```python
from build123d import *

# Parameters (mm, degrees)
CROSSRECESS_DEPTH = 2.17
FILLET5_R         = 0.3
DRAFT1_ANGLE      = -30


with BuildPart() as part:
    # Sketch1 → Base (revolve)
    with BuildSketch(Plane.XY, mode=Mode.PRIVATE) as base_sk:
        with BuildLine():
            Line((11.1, 2), (4.5, 2))
            Line((4.5, 2), (3.1, 2))
            Line((3.1, 2), (3.1, 2.35))
            Line((3.1, 2.35), (3.1, 4))
            Line((3.1, 4), (1.376524617, 4))
            ThreePointArc((1.376524617, 4), (0.353757652, 2.115113473), (0, 0))
            Line((0, 0), (11.1, 0))
            Line((11.1, 0), (11.1, 2))
        make_face()
    revolve(base_sk.sketch.rotate(Axis((4.515812911, 0, 0), (-1, 0, 0)), 90), axis=Axis((4.515812911, 0, 0), (-1, 0, 0)))

    # Sketch6 → CrossRecess (cut)
    with BuildSketch(Plane(origin=(0, 0, 0), x_dir=(0, 0, -1), z_dir=(1, 0, 0))):
        Polygon((0.44, 0.44), (0.44, 2.2), (-0.44, 2.2), (-0.44, 0.44), (-2.2, 0.44), (-2.2, -0.44), (-0.44, -0.44), (-0.44, -2.2), (0.44, -2.2), (0.44, -0.44), (2.2, -0.44), (2.2, 0.44), align=None)
    extrude(amount=CROSSRECESS_DEPTH, mode=Mode.SUBTRACT)

    # Fillet5
    fillet5_edges = [part.edges().sort_by_distance(p)[0] for p in [
        (1.099926585, 0.44, 0.44),
        (1.099926585, -0.44, 0.44),
        (1.099926585, -0.44, -0.44),
        (1.099926585, 0.44, -0.44),
    ]]
    fillet(fillet5_edges, radius=FILLET5_R)

    # Draft1
    draft1_faces = [part.faces().sort_by_distance(p)[0] for p in [
        (1.27944778, -2.2, 0),
        (1.27944778, 0, -2.2),
        (1.27944778, 0, 2.2),
        (1.27944778, 2.2, 0),
    ]]
    draft(draft1_faces, Plane(origin=(0, 0, 0), x_dir=(0, 0, 1), z_dir=(1, 0, 0)), DRAFT1_ANGLE)


solid = part.part
```
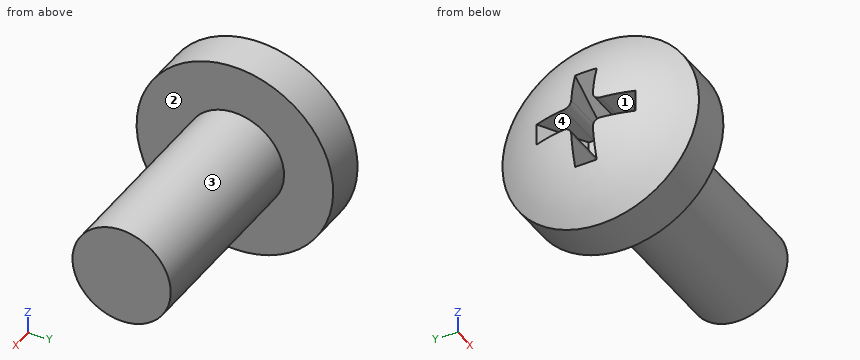
Can you work these out from the model? Positions are in its coordinate system, mm. Face numbers are marked on the shaded views. Give positions to 0.01 mm unless a question says otherwise; leave off trailing zeros. Order: outer loops, then holes, each group sorted by start corner. A loop starts at its lowest first (then second) coordinate and runs counter-clockwise, first axis right, second up. Notation, with made-up numbers: M 50.5,-12.5 L 84.5,-12.5 A24 ccw 84.5,19.5 Z; hole C -7,33 d4. An arc over 180 degrees is marked long. Write item = value, one per line. Start each with the question number.
Q1. I need wall thicknesses on probe 1 along Y at (x, z) = (7.5, 0); probe 2 along X at (y, z) = (0.5, 0); probe 3 along Z at (x, y) = (1.25, 0.5). Which ranges of each line are inside material? Lowest first, please. Write a range as [from, to].
Q2. Will these pins go through, and if not, where does the flat tip stop? pin 1 Ø1.5 at (y, z) = (3, 3) entering from +X; pin 2 Ø3 at (y, z) = (1.5, -2.5) entering from -X; pin 3 Ø0.6 at (y, z) = (-0.5, 0.5) entering from -X; pin 4 Ø1 at (x, z) = (1, 1.5) entering from -Y.
Q3. Suppose I cut it at C-C (x = 4.75). Write out the boundary of the cut face in (y, z), plus the area to 3 significant figures.
Q4. We'd pull the mould along Z, two halves only. Please class the marked faces 1, 2, 3 and 4: pulls with the +Z half, pulls with the -Z half, needs draft (parallel to the pull), parting line crosses it, or undercut.
Q5. Suppose I cut it at A-A (z = 0). Write out the boundary of the cut face in (x, y), plus the area to 3 significant figures.
Q6. Suppose I cut it at D-D (y = 3). Write out the boundary of the cut face in (x, z), plus the area to 3 significant figures.
Check result:
q1.probe_1 = [-2, 2]
q1.probe_2 = [2.17, 11.1]
q1.probe_3 = [-3.8, -0.56], [0.56, 3.8]
q2.pin_1 = 3.1
q2.pin_2 = 0.16
q2.pin_3 = 0.04
q2.pin_4 = -3.82
q3.outline = C 0,0 d4
q3.area = 12.6 mm2
q4.face_1 = undercut
q4.face_2 = needs draft
q4.face_3 = parting line crosses it
q4.face_4 = undercut
q5.outline = M 0.32,-2.02 A6.5 ccw 1.38,-4 L 3.1,-4 L 3.1,-2 L 11.1,-2 L 11.1,2 L 3.1,2 L 3.1,4 L 1.38,4 A6.5 ccw 0.32,2.02 L 2.17,0.95 L 2.17,-0.95 Z
q5.area = 47.0 mm2
q6.outline = M 1.38,-2.65 L 3.1,-2.65 L 3.1,2.65 L 1.38,2.65 A5.77 ccw Z
q6.area = 11.4 mm2
